Read the model definition and answer for the solid it produces. Units are mm, in the model's axes. A direction names the side the tool comes from. Coordinates: 2 decimals unless noted, no trailing zeros. Write each loop counter-clockwise with the first axis right and the second up, starting at its lowest first coordinate (ties: lowest second). Pieces come first, ordered by that corner, then holes.
from build123d import *

# Parameters (mm, degrees)
SKETCH1_W           = 35
SKETCH1_H           = 28.5
BOSS_EXTRUDE1_DEPTH = 25
SKETCH2_R           = 4.25
CUT_EXTRUDE1_DEPTH  = 20
SKETCH3_R           = 11.25
CUT_EXTRUDE2_DEPTH  = 7.5
SKETCH9_W           = 35
SKETCH9_H           = 5
BOSS_EXTRUDE4_DEPTH = 22
SKETCH4_W           = 4
SKETCH4_H           = 47
BOSS_EXTRUDE2_DEPTH = 20
FILLET1_R           = 1.5
CUT_EXTRUDE3_REACH  = 66.415
SKETCH6_R           = 2.15
MIRROR1_START       = -14.2
MIRROR1_OUTLINE_W   = 20
MIRROR1_OUTLINE_H   = 47
MIRROR1_OUTLINE_R   = 2.15
MIRROR1_DEPTH       = 4
MIRROR1_2_DEPTH     = 47
FILLET2_R           = 1.5
SKETCH10_R          = 2
CUT_EXTRUDE4_DEPTH  = 4.3


with BuildPart() as part:
    # Sketch1 → Boss-Extrude1 (new body)
    with BuildSketch(Plane.XY):
        with BuildLine():
            ThreePointArc((-17.5, 14.25), (0, 31.75), (17.5, 14.25))
            Line((17.5, 14.25), (-17.5, 14.25))
        make_face()
        Rectangle(SKETCH1_W, SKETCH1_H)
    extrude(amount=BOSS_EXTRUDE1_DEPTH)

    # Sketch2 → Cut-Extrude1 (cut)
    with BuildSketch(Plane.XY.offset(25)):
        with Locations((0, 9.25)):
            Circle(SKETCH2_R)
    extrude(amount=-CUT_EXTRUDE1_DEPTH, mode=Mode.SUBTRACT)

    # Sketch3 → Cut-Extrude2 (cut)
    with BuildSketch(Plane.XY.offset(25)):
        with Locations((0, 9.25)):
            Circle(SKETCH3_R)
    extrude(amount=-CUT_EXTRUDE2_DEPTH, mode=Mode.SUBTRACT)

    # Sketch9 → Boss-Extrude4 (add)
    with BuildSketch(Plane.XY.offset(25)):
        with Locations((0, -11.75)):
            Rectangle(SKETCH9_W, SKETCH9_H)
    extrude(amount=BOSS_EXTRUDE4_DEPTH)

    # Sketch4 → Boss-Extrude2 (add)
    with BuildSketch(Plane.XZ.offset(14.25)):
        with Locations((12.2, 23.5)):
            Rectangle(SKETCH4_W, SKETCH4_H)
    extrude(amount=BOSS_EXTRUDE2_DEPTH)

    # Fillet1
    fillet1_edges = [part.edges().sort_by_distance(p)[0] for p in [
        (14.2, -14.25, 23.5),
        (17.5, -14.25, 23.5),
    ]]
    fillet(fillet1_edges, radius=FILLET1_R)

    # Sketch6 → Cut-Extrude3 (cut, up to next)
    with BuildSketch(Plane.ZY.offset(-10.2), mode=Mode.PRIVATE) as cut_extrude3_sk1:
        with Locations(Location((6, -24.25, 0), (0, 0, 270))):
            Circle(SKETCH6_R)
    cut_extrude3_tool1 = extrude(cut_extrude3_sk1.sketch, amount=-CUT_EXTRUDE3_REACH, mode=Mode.PRIVATE) & part.part
    # Sketch6 → Cut-Extrude3 (cut, up to next)
    with BuildSketch(Plane.ZY.offset(-10.2), mode=Mode.PRIVATE) as cut_extrude3_sk2:
        with Locations(Location((41, -24.25, 0), (0, 0, 270))):
            Circle(SKETCH6_R)
    cut_extrude3_tool2 = extrude(cut_extrude3_sk2.sketch, amount=-CUT_EXTRUDE3_REACH, mode=Mode.PRIVATE) & part.part
    add(cut_extrude3_tool1.solids().sort_by_distance((10.2, -24.25, 6))[0], mode=Mode.SUBTRACT)
    add(cut_extrude3_tool2.solids().sort_by_distance((10.2, -24.25, 41))[0], mode=Mode.SUBTRACT)

    # Mirror1: read off the stored shape, not the designer's step
    # Mirror1 outline → Mirror1 (add)
    with BuildSketch(Plane.YZ.offset(MIRROR1_START)):
        with Locations((-24.25, 23.5)):
            Rectangle(MIRROR1_OUTLINE_W, MIRROR1_OUTLINE_H)
        with Locations((-24.25, 6)):
            Circle(MIRROR1_OUTLINE_R, mode=Mode.SUBTRACT)
        with Locations((-24.25, 41)):
            Circle(MIRROR1_OUTLINE_R, mode=Mode.SUBTRACT)
    extrude(amount=MIRROR1_DEPTH)

    # Mirror1 2 outline → Mirror1 2 (add)
    with BuildSketch(Plane.XY):
        with BuildLine():
            Line((-14.2, -14.25), (-15.7, -14.25))
            ThreePointArc((-15.7, -14.25), (-14.639339828, -14.689339828), (-14.2, -15.75))
            Line((-14.2, -15.75), (-14.2, -14.25))
        make_face()
    extrude(amount=MIRROR1_2_DEPTH)

    # Fillet2
    fillet2_edges = [part.edges().sort_by_distance(p)[0] for p in [
        (-17.5, 2.5, 25),
        (17.5, 2.5, 25),
        (-17.5, -9.25, 36),
        (0, -9.25, 25),
        (17.5, -9.25, 36),
        (-16.6, -14.25, 47),
        (14.2, -25, 47),
        (14.2, -34.25, 23.5),
        (0, 31.75, 25),
        (17.5, -11, 47),
        (15.85, -14.25, 47),
        (17.060660172, -13.810660172, 47),
        (14.639339828, -14.689339828, 47),
        (-14.2, -34.25, 23.5),
        (-14.2, -25, 47),
        (-14.639339828, -14.689339828, 47),
        (-17.5, -14.25, 23.5),
    ]]
    fillet(fillet2_edges, radius=FILLET2_R)

    # Sketch10 → Cut-Extrude4 (cut)
    with BuildSketch(Plane(origin=(0, -9.25, 0), x_dir=(1, 0, 0), z_dir=(0, 1, 0))):
        with Locations(Location((10.8, -33.5, 0), (0, 0, 270))):
            Circle(SKETCH10_R)
        with Locations(Location((-11.2, -43.7, 0), (0, 0, 270))):
            Circle(SKETCH10_R)
    extrude(amount=-CUT_EXTRUDE4_DEPTH, mode=Mode.SUBTRACT)


solid = part.part
Item 1: The part is cut by section C-C (x = 0). Give the vertices of the cut face in (y, z).
Item 2: The part is cut by section B-B (y = -24.25). Give the vertices of the cut face in (x, z), and give its area (3 significant figures).
Item 3: Determine the mould class of faces 5 (the flat face through (5, 9, 17.5)), 6 (the cylindrical face through (-12.23, -24.53, 43.13)), 7 (the cylindrical face through (17.05, -11.41, 46.57)), 8 (the cylindrical face through (10.034, -11.37, 35.347)) for opening direction X: +X half, -X half, draft (parallel to the pull), parting line (faces both ways), or undercut.
Item 4: Given pin 1 (4.5 mm diameter, centred on x = 10, z = 33.5, fed in from +Y); pin 2 (8 mm diameter, centred on y = -17.5, z = 28, fed in from -X); pin 3 (16 mm diameter, centred on y = -23, z = 22, fed in from -X); pin 4 (3.5 mm diameter, centred on y = -24.25, z = 6, fed in from +X), each flat-ended and moving along its own axis, determine where each tip first touches the part or whether it passes through.
Item 5: Find the intervals of material crossed by probe 1 along Z at (x, y) = (-11, -24); probe 2 along Y at (x, z) = (0, 11.5); probe 3 along X at (y, z) = (9, 21), in increasing order.
Item 6: The part is cut by section D-D (y = 0). Give the vertices of the cut face in (x, z).
Item 7: The part is cut by section A-A (z = 33.5). Give the vertices of the cut face in (x, y).
Item 8: For faces 1 (the flat face through (10.2, -24, 23)), 2 (the flat face through (-11, -13.55, 44)), 3 (the flat face through (0, 9, 5)), 4 (the flat face through (0, -9.25, 37)), determine the directions among +Z, -Z, +X, -X, +Y, -Y from which every point of the face is accessible in a straight line to the end or side of a thin tool.
Answer:
1. outline: (-14.25, 0) - (31.75, 0) - (31.75, 23.5) arc R1.5 ccw to (30.25, 25) - (20.5, 25) - (20.5, 17.5) - (13.5, 17.5) - (13.5, 5) - (5, 5) - (5, 17.5) - (-2, 17.5) - (-2, 25) - (-7.75, 25) arc R1.5 cw to (-9.25, 26.5) - (-9.25, 47) - (-14.25, 47) - close
2. outline: (-14.2, 0) - (-10.2, 0) - (-10.2, 3.85) - (-14.2, 3.85) - close; (-14.2, 8.15) - (-10.2, 8.15) - (-10.2, 38.85) - (-14.2, 38.85) - close; (-14.2, 43.15) - (-10.2, 43.15) - (-10.2, 47) - (-12.7, 47) arc R1.5 ccw to (-14.2, 45.5) - close; (10.2, 0) - (14.2, 0) - (14.2, 3.85) - (10.2, 3.85) - close; (10.2, 8.15) - (14.2, 8.15) - (14.2, 38.85) - (10.2, 38.85) - close; (10.2, 43.15) - (14.2, 43.15) - (14.2, 45.5) arc R1.5 ccw to (12.7, 47) - (10.2, 47) - close
2. area: 306 mm2
3. face 5: undercut
3. face 6: draft
3. face 7: +X half
3. face 8: undercut
4. pin 1: stops at y = -9.25
4. pin 2: stops at x = -17.3
4. pin 3: stops at x = -14.4
4. pin 4: passes through
5. probe 1: z = 0 to 3.86, 8.14 to 38.86, 43.14 to 47
5. probe 2: y = -14.25 to 5, 13.5 to 31.75
5. probe 3: x = -17.5 to -11.25, 11.25 to 17.5
6. outline: (-17.5, 0) - (17.5, 0) - (17.5, 23.5) arc R1.5 ccw to (16, 25) - (6.4, 25) - (6.4, 17.5) - (-6.4, 17.5) - (-6.4, 25) - (-16, 25) arc R1.5 ccw to (-17.5, 23.5) - close
7. outline: (-17.5, -12.75) arc R1.5 ccw to (-16, -14.25) - (-15.7, -14.25) arc R1.5 cw to (-14.2, -15.75) - (-14.2, -32.75) arc R1.5 ccw to (-12.7, -34.25) - (-10.2, -34.25) - (-10.2, -14.25) - (10.2, -14.25) - (10.2, -34.25) - (12.7, -34.25) arc R1.5 ccw to (14.2, -32.75) - (14.2, -15.75) arc R1.5 cw to (15.7, -14.25) - (16, -14.25) arc R1.5 ccw to (17.5, -12.75) - (17.5, -10.75) arc R1.5 ccw to (16, -9.25) - (12.8, -9.25) - (12.8, -13.55) - (8.8, -13.55) - (8.8, -9.25) - (-16, -9.25) arc R1.5 ccw to (-17.5, -10.75) - close
8. face 1: +Z, -Z, -Y
8. face 2: +Y
8. face 3: +Z
8. face 4: +Z, +X, -X, +Y
